Can you work these out from the drawing? Everything is in mm from the part's minimum corner. Coordinates: 2 decimals unless noted, no trailing zeros. Loops run counter-clockwise (first coordinate to the right, second up) from the corner with the lowest first, then second, coordinate; pieces in that order, holes last.
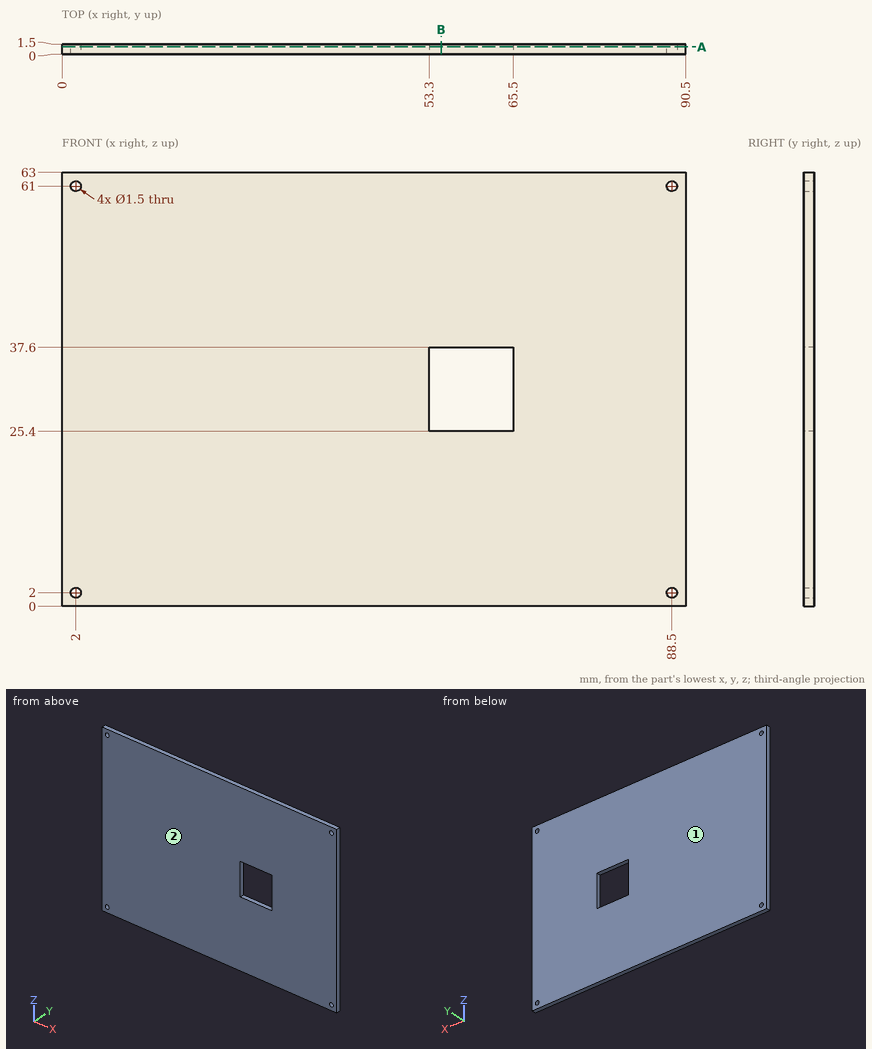
(1) For pin 1 (1.2 mm diameter, centred on x = 88.5, z = 2, fed in from -Y), with a flat end and sliding along its axis, tell me the tip position at first contact or that it passes through.
Answers:
pin 1: passes through
(2) Imagine slicing it at B-B, the plane x = 55. Write out the boundary of the cut face in (y, z).
Answers:
outline: (0, 0) - (1.5, 0) - (1.5, 25.4) - (0, 25.4) - close; (0, 37.6) - (1.5, 37.6) - (1.5, 63) - (0, 63) - close
(3) Imagine slicing it at A-A, the plane y = 1.1. Write out the boundary of the cut face in (x, z).
Answers:
outline: (0, 0) - (90.5, 0) - (90.5, 63) - (0, 63) - close; hole circle Ø1.5 at (2, 2); hole circle Ø1.5 at (2, 61); hole (53.3, 25.4) - (65.5, 25.4) - (65.5, 37.6) - (53.3, 37.6) - close; hole circle Ø1.5 at (88.5, 2); hole circle Ø1.5 at (88.5, 61)
(4) I need wall thicknesses on probe 1 along X at (y, z) = (1.15, 61); probe 2 along Z at (x, y) = (2, 0.8); probe 3 along X at (y, z) = (0.55, 26.5). Which ranges of each line are inside material? Lowest first, please.
Answers:
probe 1: x = 0 to 1.25, 2.75 to 87.75, 89.25 to 90.5
probe 2: z = 0 to 1.25, 2.75 to 60.25, 61.75 to 63
probe 3: x = 0 to 53.3, 65.5 to 90.5
(5) We'd pull the mould along Y, two halves only. Please class the marked faces 1 and 2: +Y half, -Y half, draft (parallel to the pull), parting line (faces both ways), or undercut.
Answers:
face 1: +Y half
face 2: -Y half
